Input: part model. Units: mm. Frame: model coordinates. Round coordinates to 2 decimals unless told otherwise and drop trailing zeros. Order: outer loops, then holes, each group sorted by start corner. A loop starts at its lowest first (then second) coordinate and runs counter-clockwise, first axis right, second up. Notation, with made-up numbers: (68.5, 83) -> (92.5, 83) arc R16 ccw to (92.5, 110) -> close; hole circle Ø2 at (-31.5, 58). An arc over 180 degrees is marked (long way). Use a Markdown table: item, result.
Autodesk Inventor part; units mm, degrees
ref_plane "Work Plane1" through (0, 0, 0) normal (0, 0, 1) x (1, 0, 0)
ref_plane "YZ Plane" through (0, 0, 0) normal (1, 0, 0) x (0, 1, 0)
ref_plane "XZ Plane" through (0, 0, 0) normal (0, 1, 0) x (-1, 0, 0)
ref_plane "Work Plane1" through (0, 0, 0) normal (0, 0, 1) x (1, 0, 0)
sketch "Sketch2" plane through (0, 0, 0) normal (0, 0, 1) x (1, 0, 0)
  arc A0 (-2.0996, 1.5875) -> (1.4502, 1.5875) centre (-0.3247, 0) ccw
  circle A1 centre (-0.3247, 0) radius 2.3813
  circle A2 centre (-0.3247, 0) radius 3.9633
extrude "Extrusion1" add sketch "Sketch2" along normal blind 0.7937
chamfer "Chamfer1" distance 0.127 angle 45 4 edges at (-4.288, 0, 0) (-4.288, 0, 0.7937) (-2.706, 0, 0.7937) (-2.706, 0, 0)
properties part number "thrust washer" material "Rubber"
1) Draft query along Y for faces 1 (the face through (-0.25, -2.38, 0.39)), 2 (the face through (3.456, -1.19, 0.393)), 3 (the face through (0, -3, 0)). Return one class per face: released by +Y, released by -Y, zero draft, split by the parting line, or undercut.
Answer key:
| item | result |
|---|---|
| face 1 | undercut |
| face 2 | split by the parting line |
| face 3 | zero draft |
2) Cut plane A-A on y = 0. Return loops of the section in (x, z).
Answer key:
| item | result |
|---|---|
| outline | (-4.29, 0.13) -> (-4.16, 0) -> (-2.83, 0) -> (-2.71, 0.13) -> (-2.71, 0.67) -> (-2.83, 0.79) -> (-4.16, 0.79) -> (-4.29, 0.67) -> close; (2.06, 0.13) -> (2.18, 0) -> (3.51, 0) -> (3.64, 0.13) -> (3.64, 0.67) -> (3.51, 0.79) -> (2.18, 0.79) -> (2.06, 0.67) -> close |
3) Contact query for a flat-ended pin moving along its axis: P1, Ø3, axis at x = 2.5, y = 1, coming from the -Z side. Output: stop coordinate, or through.
Answer key:
| item | result |
|---|---|
| P1 | stops at z = 0 |
4) Ray query, probe 1 along Y at (x, z) = (-2.25, 0.45); probe 2 along Y at (x, z) = (-2.5, 0.3); probe 3 along X at (y, z) = (2, 0.45). Return the intervals inside material, ascending.
Answer key:
| item | result |
|---|---|
| probe 1 | y = -3.46 to -1.4, 1.4 to 3.46 |
| probe 2 | y = -3.31 to -0.97, 0.97 to 3.31 |
| probe 3 | x = -3.75 to -1.62, 0.97 to 3.1 |
5) Cut plane B-B on z = 0.4. Return loops of the section in (x, y).
Answer key:
| item | result |
|---|---|
| outline | circle Ø7.93 at (-0.32, 0); hole circle Ø4.76 at (-0.32, 0) |
